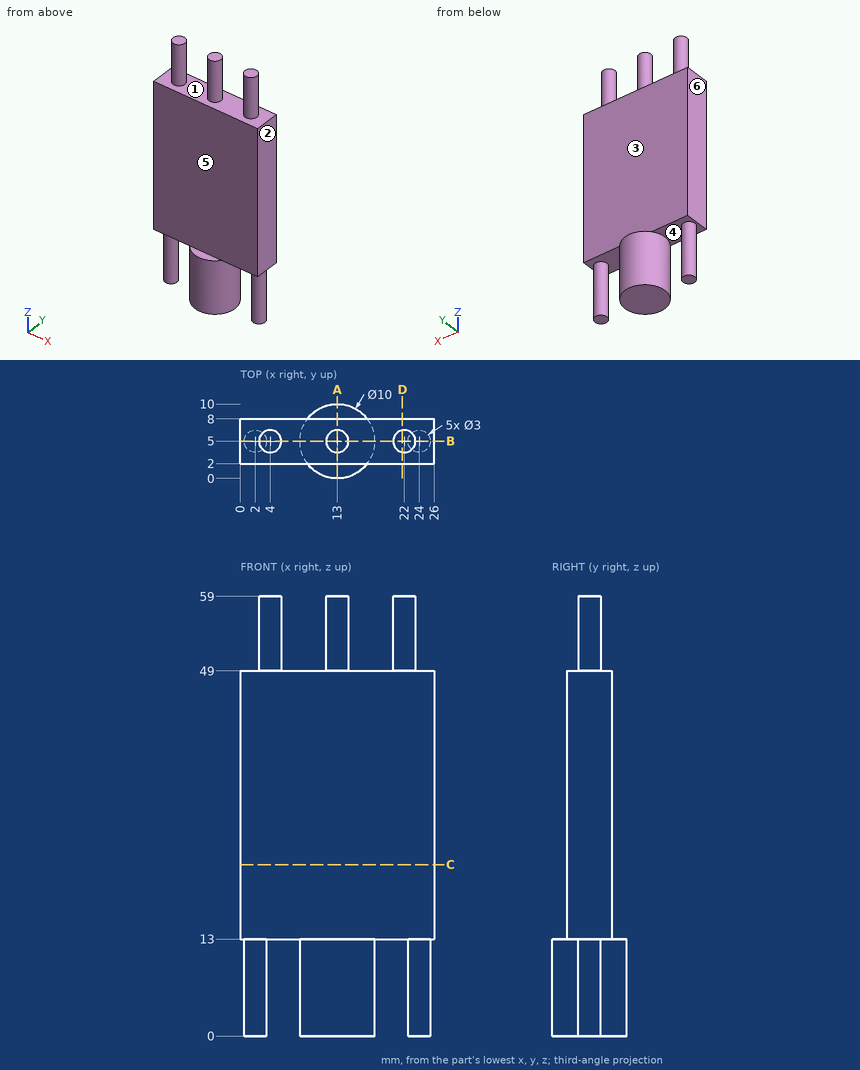
Here's the drawing with two shaded views (mm, measured from the low corner). I have some questions. A direction names the side the tool comes from. Coordinates: 2 decimals unless noted, no trailing zeros. Loops run counter-clockwise (first coordinate to the right, second up) from the corner with the lowest first, then second, coordinate; pieces in that order, holes last. Notation, with made-up numbers: (8, -24.75) -> (55, -24.75) arc R30 cw to (55, 9.25) -> close; hole circle Ø11 at (68, 74.5). An arc over 180 degrees is marked (long way). Put each result on its own line as item: value. Start each with the question number.
Q1. I want a section at D-D (x = 21.75). Write out the boundary of the cut face in (y, z).
Q2. I want a section at B-B (y = 5). Write out the boundary of the cut face in (x, z).
Q3. Thinking about a two-plate mould opening in X: for the marked faces 1, 2 and 3, which applies, pulls with the +X half, pulls with the -X half, needs draft (parallel to the pull), parting line crosses it, or undercut?
Q4. I'm going to push flat-ended pins straight in: P1, Ø2, axis at x = 3.5, y = 8.5, coming from the +Z side; P2, Ø10, axis at x = 9, z = 17, coming from the +Y side; P3, Ø3, axis at x = 11.5, z = 36.5, coming from the -Y side. Where does each tip first touch, or does it pass through?
Q5. I want a section at A-A (x = 13). Write out the boundary of the cut face in (y, z).
Q6. If I drill on line 1 (X direction, y = 6, z = 53.5); line 2 (Z direction, x = 18.75, y = 4.25); line 3 (Y direction, x = 22.5, z = 45), over which ranges is the centre line in solid material (lowest first)? Write a range as [from, to].
Q7. For the marked faces 4, 5 and 6, which set-ups out of +Z, -Z, +X, -X, +Y, -Y let a thin tool reach every point of the face, with its end or its side?
Q8. I want a section at C-C (z = 23). Write out the boundary of the cut face in (x, y), plus the area to 3 significant figures.
Taken from the geometry:
1. outline: (2, 13) -> (8, 13) -> (8, 49) -> (6.48, 49) -> (6.48, 59) -> (3.52, 59) -> (3.52, 49) -> (2, 49) -> close
2. outline: (0, 13) -> (0.5, 13) -> (0.5, 0) -> (3.5, 0) -> (3.5, 13) -> (8, 13) -> (8, 0) -> (18, 0) -> (18, 13) -> (22.5, 13) -> (22.5, 0) -> (25.5, 0) -> (25.5, 13) -> (26, 13) -> (26, 49) -> (23.5, 49) -> (23.5, 59) -> (20.5, 59) -> (20.5, 49) -> (14.5, 49) -> (14.5, 59) -> (11.5, 59) -> (11.5, 49) -> (5.5, 49) -> (5.5, 59) -> (2.5, 59) -> (2.5, 49) -> (0, 49) -> close
3. face 1: undercut
3. face 2: pulls with the +X half
3. face 3: needs draft
4. P1: stops at z = 49
4. P2: stops at y = 9.9
4. P3: stops at y = 2
5. outline: (0, 0) -> (10, 0) -> (10, 13) -> (8, 13) -> (8, 49) -> (6.5, 49) -> (6.5, 59) -> (3.5, 59) -> (3.5, 49) -> (2, 49) -> (2, 13) -> (0, 13) -> close
6. line 1: x = [2.88, 5.12], [11.88, 14.12], [20.88, 23.12]
6. line 2: z = [13, 49]
6. line 3: y = [2, 8]
7. face 4: -Z
7. face 5: +Z, +X, -X, -Y
7. face 6: +Z, -Z, -X, +Y, -Y
8. outline: (0, 2) -> (26, 2) -> (26, 8) -> (0, 8) -> close
8. area: 156 mm2
